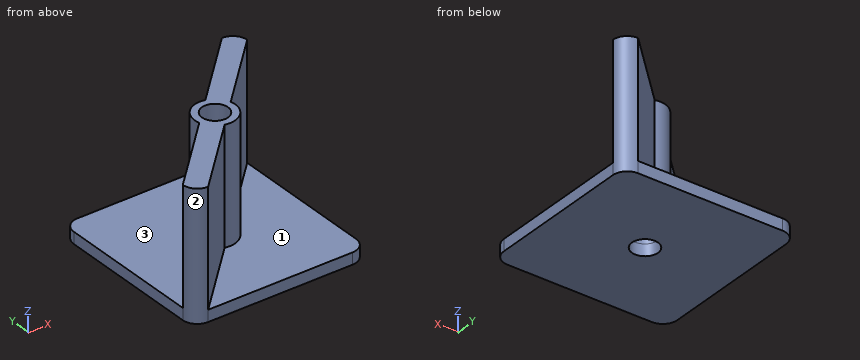
from build123d import *

# Parameters (mm, degrees)
F1_DEPTH = 4
F2_R     = 4.5
F3_DEPTH = 40
F4_DEPTH = 25


with BuildPart() as f1:
    # F0 (on Top) → F1 (new body)
    with BuildSketch(Plane.XY):
        with BuildLine():
            Line((-25, -30), (25, -30))
            ThreePointArc((25, -30), (28.535534, -28.535534), (30, -25))
            Line((30, -25), (30, 25))
            ThreePointArc((30, 25), (28.535534, 28.535534), (25, 30))
            Line((25, 30), (-25, 30))
            ThreePointArc((-25, 30), (-28.535534, 28.535534), (-30, 25))
            Line((-30, 25), (-30, -25))
            ThreePointArc((-30, -25), (-28.535534, -28.535534), (-25, -30))
        make_face()
    extrude(amount=F1_DEPTH)

    # F2 (on face) → F3 (join)
    with BuildSketch(Plane.XY.offset(4)):
        with BuildLine():
            Line((25, 30), (1.772002, 6.772002))
            ThreePointArc((1.772002, 6.772002), (-4.949747, 4.949747), (-6.772002, -1.772002))
            Line((-6.772002, -1.772002), (-30, -25))
            ThreePointArc((-30, -25), (-28.535534, -28.535534), (-25, -30))
            Line((-25, -30), (-1.772002, -6.772002))
            ThreePointArc((-1.772002, -6.772002), (4.949747, -4.949747), (6.772002, 1.772002))
            Line((6.772002, 1.772002), (30, 25))
            ThreePointArc((30, 25), (28.535534, 28.535534), (25, 30))
        make_face()
        Circle(F2_R, mode=Mode.SUBTRACT)
    extrude(amount=F3_DEPTH)

    # F2 (on face) → F4 (cut)
    with BuildSketch(Plane.XY.offset(4)):
        Circle(F2_R)
    extrude(amount=-F4_DEPTH, mode=Mode.SUBTRACT)


solid = f1.part
Geometry check sheet. Reference: the model listing, model coordinates, mm. Face numbers are marked on the shaded views. A direction names the side the tool comes from. Coordinates: 2 decimals unless noted, no trailing zeros. Loops run counter-clockwise (first coordinate to the right, second up) from the corner with the lowest first, then second, coordinate; pieces in that order, holes last. Notation, with made-up numbers: (-3.75, 42) - (2.25, 42) arc R9 ccw to (2.25, 52) - close; hole circle Ø1 at (78.25, 84). An arc over 180 degrees is marked (long way). Use one line per item in the form item = value. Start each with the question number.
Item 1: Section check D-D, the plane y = -17. Enter the section's corners in (x, z), and give its area (3 significant figures).
Item 2: Tool access check on the marked faces 1, 2 and 3. Record the directions out of +Z, -Z, +X, -X, +Y, -Y that give a thin tool (end or side, any length) a straight path to the whole face; none if there is none.
Item 3: Section check C-C, the plane z = 5.5. Enter the section's corners in (x, y), and give its area (3 significant figures).
Item 4: Gauge pin test, flat ends, axial feed: pin 1 (8 mm diameter, centred on y = 17, z = 20.5, fed in from +X); pin 2 (3 mm diameter, centred on y = 12, z = 37.5, fed in from -X); pin 3 (10 mm diameter, centred on y = -1, z = 11.5, fed in from -X). Record the tip position at first contact, or that the pin passes through.
Item 5: Section check A-A, the plane x = 0. Enter the section's corners in (y, z), and give its area (3 significant figures).
Item 6: Thickness scan on probe 1 along Y at (x, z) = (0, 15); probe 2 along Y at (x, z) = (0, 1.85); probe 3 along Z at (x, y) = (-11.5, 1). Record the ranges inside material, lowest first.
Computed:
q1.outline = (-30, 0) - (30, 0) - (30, 4) - (-12, 4) - (-12, 44) - (-22, 44) - (-22, 4) - (-30, 4) - close
q1.area = 640 mm2
q2.face_1 = +Z, +X, -Y
q2.face_2 = +Z, -Z, -X, -Y
q2.face_3 = +Z, -X, +Y
q3.outline = (-30, -25) arc R5 ccw to (-25, -30) - (-1.77, -6.77) arc R7 ccw to (6.77, 1.77) - (30, 25) arc R5 ccw to (25, 30) - (1.77, 6.77) arc R7 ccw to (-6.77, -1.77) - close; hole circle Ø9 at (0, 0)
q3.area = 560 mm2
q4.pin_1 = 26
q4.pin_2 = 5.5
q4.pin_3 = -11
q5.outline = (-30, 0) - (-4.5, 0) - (-4.5, 44) - (-7, 44) - (-7, 4) - (-30, 4) - close; (4.5, 0) - (30, 0) - (30, 4) - (7, 4) - (7, 44) - (4.5, 44) - close
q5.area = 404 mm2
q6.probe_1 = -7 to -4.5, 4.5 to 7
q6.probe_2 = -30 to -4.5, 4.5 to 30
q6.probe_3 = 0 to 4
